```python
from build123d import *

# Parameters (mm, degrees)
SKETCH1_W                  = 120
SKETCH1_H                  = 120
BOSS_EXTRUDE1_DEPTH        = 5
F_3_3_3_3_DIAMETER_HOLE1_D = 3.3
SKETCH5_W                  = 5.1
SKETCH5_H                  = 5
SKETCH5_W_2                = 5
SKETCH5_H_2                = 5.1
CUT_EXTRUDE1_DEPTH         = 6


with BuildPart() as part:
    # Sketch1 → Boss-Extrude1 (new body)
    with BuildSketch(Plane(origin=(0, 0, 0), x_dir=(1, 0, 0), z_dir=(0, 1, 0))):
        Rectangle(SKETCH1_W, SKETCH1_H)
    extrude(amount=BOSS_EXTRUDE1_DEPTH)

    # Ø3.3 (3.3) Diameter Hole1 (through all)
    with Locations(Plane(origin=(0, 5, 0), x_dir=(1, 0, 0), z_dir=(0, 1, 0))):
        with Locations((-45, 45), (45, 45), (45, -45), (-45, -45)):
            Hole(F_3_3_3_3_DIAMETER_HOLE1_D / 2)

    # Sketch5 → Cut-Extrude1 (cut, through all)
    with BuildSketch(Plane(origin=(0, 5, 0), x_dir=(1, 0, 0), z_dir=(0, 1, 0))):
        with Locations((-55.45, 50)):
            Rectangle(SKETCH5_W, SKETCH5_H)
        with Locations((-55.45, -50)):
            Rectangle(SKETCH5_W, SKETCH5_H)
        with Locations((-50, -55.45)):
            Rectangle(SKETCH5_W_2, SKETCH5_H_2)
        with Locations((50, -55.45)):
            Rectangle(SKETCH5_W_2, SKETCH5_H_2)
        with Locations((-50, 55.45)):
            Rectangle(SKETCH5_W_2, SKETCH5_H_2)
        with Locations((50, 55.45)):
            Rectangle(SKETCH5_W_2, SKETCH5_H_2)
        with Locations((55.45, 50)):
            Rectangle(SKETCH5_W, SKETCH5_H)
        with Locations((55.45, -50)):
            Rectangle(SKETCH5_W, SKETCH5_H)
        with Locations((-55.45, 0)):
            Rectangle(SKETCH5_W, SKETCH5_H)
        with Locations((0, 55.45)):
            Rectangle(SKETCH5_W_2, SKETCH5_H_2)
        with Locations((0, -55.45)):
            Rectangle(SKETCH5_W_2, SKETCH5_H_2)
        with Locations((55.45, 0)):
            Rectangle(SKETCH5_W, SKETCH5_H)
    extrude(amount=-CUT_EXTRUDE1_DEPTH, mode=Mode.SUBTRACT)


solid = part.part
```
Model file for the job. Use its own axes, mm. Round coordinates to 2 decimals unless told otherwise and drop trailing zeros. Loops run counter-clockwise (first coordinate to the right, second up) from the corner with the lowest first, then second, coordinate; pieces in that order, holes last. Notation, with made-up numbers: M 79.25,47.5 L 117.25,47.5 A35 ccw 117.25,82.5 Z; hole C -40,-21.75 d11. An arc over 180 degrees is marked long. Put each result on its own line as item: value. Start each with the question number.
Item 1: Cut at A-A (z = 0). List the corners of the cut face in (x, y), then the cut area to 3 significant figures.
Item 2: Mould opens along Z. For faces 1 (the face through (-1, 5, -1)), 2 (the face through (0, 3, 52.9)) say: released by +Z, released by -Z, zero draft, split by the parting line, or undercut.
Item 3: Cut at B-B (x = -50.5). List the corners of the cut face in (y, z), then the cut area to 3 significant figures.
Item 4: Cut at C-C (y = 1.5). Give the number of separate pieces and of enclosed holes in the cut face, then the cut area to 3 significant figures.
Item 5: Drill centre lines: line 1 along Z through (x, y) = (-48.5, 3.9); line 2 along Z through (x, y) = (45, 2.25). Where is each one in solid material? Low to high.
Answer block:
1. outline: M -60,0 L -58,0 L -58,5 L -60,5 Z; M -52.9,0 L 52.9,0 L 52.9,5 L -52.9,5 Z; M 58,0 L 60,0 L 60,5 L 58,5 Z
1. area: 549 mm2
2. face 1: zero draft
2. face 2: undercut
3. outline: M 0,-60 L 5,-60 L 5,-58 L 0,-58 Z; M 0,-52.9 L 5,-52.9 L 5,52.9 L 0,52.9 Z; M 0,58 L 5,58 L 5,60 L 0,60 Z
3. area: 549 mm2
4. separate pieces: 1
4. enclosed holes: 16
4. area: 14,100 mm2
5. line 1: -60 to -58, -52.9 to 52.9, 58 to 60
5. line 2: -60 to -46.65, -43.35 to 43.35, 46.65 to 60
